```python
from build123d import *

# Parameters (mm, degrees)
BOSS_EXTRUDE1_DEPTH = 125
SKETCH4_R           = 9
CUT_EXTRUDE1_DEPTH  = 152.817765536
SKETCH5_R           = 9
CUT_EXTRUDE2_DEPTH  = 154.447072098


with BuildPart() as part:
    # Sketch1 → Boss-Extrude1 (new body)
    with BuildSketch(Plane(origin=(0, 0, 0), x_dir=(1, 0, 0), z_dir=(0, 1, 0))):
        Polygon((-78.284726088, 35.987992356), (-78.284726088, 29.637992356), (-33.284726088, 29.637992356), (14.724277299, -6.35), (59.724277299, -6.35), (59.724277299, 0), (14.724277299, 0), (-33.284726088, 35.987992356), align=None)
    extrude(amount=BOSS_EXTRUDE1_DEPTH)

    # Sketch4 → Cut-Extrude1 (cut, through all)
    with BuildSketch(Plane.XY.offset(-29.637992356)):
        with Locations((-55.784726088, 95)):
            Circle(SKETCH4_R)
        with Locations((-55.784726088, 32)):
            Circle(SKETCH4_R)
    extrude(amount=-CUT_EXTRUDE1_DEPTH, mode=Mode.SUBTRACT)

    # Sketch5 → Cut-Extrude2 (cut, through all)
    with BuildSketch(Plane.XY.offset(6.35)):
        with Locations((37.224277299, 95)):
            Circle(SKETCH5_R)
        with Locations((37.224277299, 32)):
            Circle(SKETCH5_R)
    extrude(amount=-CUT_EXTRUDE2_DEPTH, mode=Mode.SUBTRACT)


solid = part.part
```
CAD build for the part. Positions are in the model's coordinates, mm. A direction names the side the tool comes from. Round coordinates to 2 decimals unless told otherwise and drop trailing zeros. Loops run counter-clockwise (first coordinate to the right, second up) from the corner with the lowest first, then second, coordinate; pieces in that order, holes last. Notation, with made-up numbers: (40, -36.5) - (50, -36.5) arc R12 ccw to (50, -18.5) - close; hole circle Ø10 at (76.5, 70). An arc over 180 degrees is marked (long way). Return JSON: item names as keys, results as strings. Group by question number.
Q1. Band-saw the part on D-D on x = -41.5. Give the cut face in (y, z), plus the area to 3 significant figures.
Q2. Band-saw the part on C-C on z = -32. Give the cut face in (x, y).
Q3. Band-saw the part on A-A on y = 32. Give the cut face in (x, z), plus the area to 3 significant figures.
Q4. Flat gauge pins, fed straight in: pin 1 Ø12 at (x, y) = (-55, 21.5) entering from +Z; pin 2 Ø10 at (x, y) = (0, 25.5) entering from +Z; pin 3 Ø5 at (x, y) = (-30, 23.5) entering from +Z; pin 4 Ø16 at (x, y) = (37.22, 95) entering from -Z. Where does each tip first touch, or does it go through?
Q5. Band-saw the part on B-B on y = 11. Give the cut face in (x, z), plus the area to 3 significant figures.
Q6. Tool access for faces 1 (the face through (-56, 62, -29.638)), 2 (the face through (38, 62, 0)), 3 (the face through (-57.736, 86.214, -32.769)): list every direction of +Z, -Z, +X, -X, +Y, -Y with a clear straight run to the whole face (end or side of a thin tool).
Q7. Drill centre lines: line 1 along Z through (x, y) = (37, 79); line 2 along Y through (x, z) = (-57.5, -30.5); line 3 along Z through (x, y) = (-45, 59). Where is each one in solid material? Low to high. Write a range as [from, to].
Solutions:
{
 "1": {"outline": "(0, -35.99) - (125, -35.99) - (125, -29.64) - (0, -29.64) - close", "area": "794 mm^2"},
 "2": {"outline": "(-78.28, 0) - (-27.96, 0) - (-27.96, 125) - (-78.28, 125) - close; hole circle Ø18 at (-55.78, 32); hole circle Ø18 at (-55.78, 95)"},
 "3": {"outline": "(-78.28, -35.99) - (-64.78, -35.99) - (-64.78, -29.64) - (-78.28, -29.64) - close; (-46.78, -35.99) - (-33.28, -35.99) - (14.72, 0) - (28.22, 0) - (28.22, 6.35) - (14.72, 6.35) - (-33.28, -29.64) - (-46.78, -29.64) - close; (46.22, 0) - (59.72, 0) - (59.72, 6.35) - (46.22, 6.35) - close", "area": "648 mm^2"},
 "4": {"pin 1": "stops at z = -29.64", "pin 2": "stops at z = -0.94", "pin 3": "stops at z = -25.3", "pin 4": "passes through"},
 "5": {"outline": "(-78.28, -35.99) - (-33.28, -35.99) - (14.72, 0) - (59.72, 0) - (59.72, 6.35) - (14.72, 6.35) - (-33.28, -29.64) - (-78.28, -29.64) - close", "area": "876 mm^2"},
 "6": {"face 1": "+Z, -X, +Y, -Y", "face 2": "-Z, +X, +Y, -Y", "face 3": "+Z, -Z"},
 "7": {"line 1": "z = [0, 6.35]", "line 2": "y = [0, 23.16], [40.84, 86.16], [103.84, 125]", "line 3": "z = [-35.99, -29.64]"}
}
